Geometry: final body of the model. Coordinates: model frame, mm. A direction names the side the tool comes from. Round coordinates to 2 decimals unless told otherwise and drop trailing zeros. Write each loop counter-clockwise with the first axis right and the second up, starting at its lowest first coordinate (ties: lowest second). Pieces come first, ordered by that corner, then holes. Notation, with made-up numbers: M -39,4 L -17,4 A16 cw -17,31 Z; hole C 78,34.5 d10. An arc over 180 degrees is marked long. Answer as CSV lines item,"result". Start each with the question number.
Q1. Section query A-A on y = 23. Output: boundary loops of the cut face in (x, z).
Q2. First-contact query: pin 1 (5 mm diameter, centred on x = 82.5, y = 7.5, fed in from +Z); pin 2 (5 mm diameter, centred on x = 37.5, z = 6.5, fed in from +Y); pin 3 (1 mm diameter, centred on y = 12.5, z = 4, fed in from -X); pin 4 (4.5 mm diameter, centred on x = 67, z = 5.5, fed in from +Y). Flat tips, straight axial feed; report the tip coordinate or a pass-through.
Q3. Section query B-B on z = 8. Give the number of separate pieces and of enclosed holes in the cut face, and give its area (3 significant figures).
Q4. Section query D-D on y = 58. Output: boundary loops of the cut face in (x, z), and give its area (3 significant figures).
Q5. Reachability of faces 1 (the cylindrical face through (1.203, 66.859, 4.437)), 2 (the flat face through (8, 28, 5)), 3 (the flat face through (70, 44, 5)) from +Z, -Z, +X, -X, +Y, -Y: full face, straight path, thin tool, end or side. Return the list, or none.
Q6. Mould query, pull axis Y, two halves, no side actions, for faces 4 (the cylindrical face through (58.27, 16.31, 4.56)), 5 (the flat face through (42, 56, 5)), 6 (the cylindrical face through (13.39, 27.69, 4.44)). Classes: pulls with the +Y half, pulls with the -Y half, needs draft (parallel to the pull), parting line crosses it, or undercut.
Q7. Section query C-C on x = 51.5. Output: boundary loops of the cut face in (y, z), and give its area (4 significant figures).
Q8. Ray query, probe 1 along Y at (x, z) = (5, 2.75); probe 2 along Y at (x, z) = (67, 5.25); probe 3 along Y at (x, z) = (82.5, 6). Return the intervals inside material, ascending.
```python
from build123d import *

# Parameters (mm, degrees)
ESQUISSE1_W             = 88
ESQUISSE1_H             = 96
BOSS_EXTRU_1_DEPTH      = 9
ESQUISSE2_R             = 2
ENL_V_MAT_EXTRU_1_DEPTH = 131.541181242
ESQUISSE3_R             = 1.5
ESQUISSE3_R_2           = 11
ENL_V_MAT_EXTRU_2_DEPTH = 131.541181242
ESQUISSE4_W             = 88
ESQUISSE4_H             = 28
ENL_V_MAT_EXTRU_3_DEPTH = 131.541181242
ENL_V_MAT_EXTRU_4_DEPTH = 9
ESQUISSE6_W             = 41.5
ESQUISSE6_H             = 28
ENL_V_MAT_EXTRU_5_DEPTH = 112.575086825
ESQUISSE7_W             = 46.5
ESQUISSE7_H             = 2
ENL_V_MAT_EXTRU_6_DEPTH = 112.575086825
CHANFREIN1_SIZE         = 28
CONG_1_R                = 4


with BuildPart() as part:
    # Esquisse1 → Boss.-Extru.1 (new body)
    with BuildSketch(Plane.XY):
        with Locations((44, 48)):
            Rectangle(ESQUISSE1_W, ESQUISSE1_H)
    extrude(amount=BOSS_EXTRU_1_DEPTH)

    # Esquisse2 → Enlèv. mat.-Extru.1 (cut, through all)
    with BuildSketch(Plane.XY.offset(9)):
        with Locations((5, 58)):
            Circle(ESQUISSE2_R)
        with Locations(Location((5, 38, 0), (0, 0, 180))):
            Circle(ESQUISSE2_R)
        with Locations((25, 38)):
            Circle(ESQUISSE2_R)
        with Locations(Location((25, 58, 0), (0, 0, 180))):
            Circle(ESQUISSE2_R)
    extrude(amount=-ENL_V_MAT_EXTRU_1_DEPTH, mode=Mode.SUBTRACT)

    # Esquisse3 → Enlèv. mat.-Extru.2 (cut, through all)
    with BuildSketch(Plane.XY.offset(9)):
        with Locations((82.5, 38.5)):
            Circle(ESQUISSE3_R)
        with Locations(Location((82.5, 7.5, 0), (0, 0, 180))):
            Circle(ESQUISSE3_R)
        with Locations((51.5, 7.5)):
            Circle(ESQUISSE3_R)
        with Locations(Location((51.5, 38.5, 0), (0, 0, 180))):
            Circle(ESQUISSE3_R)
        with Locations((67, 23)):
            Circle(ESQUISSE3_R_2)
    extrude(amount=-ENL_V_MAT_EXTRU_2_DEPTH, mode=Mode.SUBTRACT)

    # Esquisse4 → Enlèv. mat.-Extru.3 (cut, through all)
    with BuildSketch(Plane.XY.offset(9)):
        with Locations((44, 82)):
            Rectangle(ESQUISSE4_W, ESQUISSE4_H)
    extrude(amount=-ENL_V_MAT_EXTRU_3_DEPTH, mode=Mode.SUBTRACT)

    # Esquisse5 → Enlèv. mat.-Extru.4 (cut)
    with BuildSketch(Plane.XY.offset(9)):
        Polygon((30, 68), (54, 44), (88, 44), (88, 68), align=None)
    extrude(amount=-ENL_V_MAT_EXTRU_4_DEPTH, mode=Mode.SUBTRACT)

    # Esquisse6 → Enlèv. mat.-Extru.5 (cut, through all)
    with BuildSketch(Plane.XY.offset(9)):
        with Locations((20.75, 14)):
            Rectangle(ESQUISSE6_W, ESQUISSE6_H)
    extrude(amount=-ENL_V_MAT_EXTRU_5_DEPTH, mode=Mode.SUBTRACT)

    # Esquisse7 → Enlèv. mat.-Extru.6 (cut, through all)
    with BuildSketch(Plane.XY.offset(9)):
        with Locations((64.75, 1)):
            Rectangle(ESQUISSE7_W, ESQUISSE7_H)
    extrude(amount=-ENL_V_MAT_EXTRU_6_DEPTH, mode=Mode.SUBTRACT)

    # Chanfrein1
    # the kernel refuses this chamfer: 28 mm, written as the material it adds along each edge
    with BuildSketch(Plane(origin=(41.5, 28, 9), x_dir=(0.027495876610586358, -0.9996219169112968, 0), z_dir=(0, 0, -1))) as chanfrein1_piece_1_section:
        Polygon((CHANFREIN1_SIZE * 0.999621916911, CHANFREIN1_SIZE * 0.0274958766106), (-CHANFREIN1_SIZE * 0.0274958766106, CHANFREIN1_SIZE * 0.999621916911), (0, 0), align=None)
    chanfrein1_piece_1 = extrude(amount=9, mode=Mode.PRIVATE)
    chanfrein1_piece_1 = split(chanfrein1_piece_1, bisect_by=Plane(origin=(32.152400719, 2, 4.5), z_dir=(0, 1, 0)), keep=Keep.TOP, mode=Mode.PRIVATE)
    add(chanfrein1_piece_1)

    # Congé1
    cong_1_edges = [part.edges().sort_by_distance(p)[0] for p in [
        (88, 2, 4.5),
        (13.5, 28, 4.5),
        (39.5, 2, 4.5),
        (0, 68, 4.5),
        (30, 68, 4.5),
        (88, 44, 4.5),
        (54, 44, 4.5),
        (0, 28, 4.5),
    ]]
    fillet(cong_1_edges, radius=CONG_1_R)


solid = part.part
```
Entries:
1,outline,"M 18.5,0 L 56,0 L 56,9 L 18.5,9 Z; M 78,0 L 88,0 L 88,9 L 78,9 Z"
2,pin 1,"stops at z = 9"
2,pin 2,"stops at y = 63"
2,pin 3,"stops at x = 28.5"
2,pin 4,"stops at y = 44"
3,separate pieces,"1"
3,enclosed holes,"9"
3,area,"3,540 mm^2"
4,outline,"M 0,0 L 3,0 L 3,9 L 0,9 Z; M 7,0 L 23,0 L 23,9 L 7,9 Z; M 27,0 L 40,0 L 40,9 L 27,9 Z"
4,area,"288 mm^2"
5,face 1,"+Z, -Z, -X, +Y"
5,face 2,"+Z, -Z, -X, -Y"
5,face 3,"+Z, -Z, +X, +Y"
6,face 4,"undercut"
6,face 5,"pulls with the +Y half"
6,face 6,"pulls with the -Y half"
7,outline,"M 2,0 L 6,0 L 6,9 L 2,9 Z; M 9,0 L 37,0 L 37,9 L 9,9 Z; M 40,0 L 46.5,0 L 46.5,9 L 40,9 Z"
7,area,"346.5 mm^2"
8,probe 1,"y = 28 to 36, 40 to 56, 60 to 68"
8,probe 2,"y = 2 to 12, 34 to 44"
8,probe 3,"y = 2 to 6, 9 to 37, 40 to 44"
